```python
from build123d import *

# Parameters (mm, degrees)
CROQUIS1_R              = 3
SALIENTE_EXTRUIR1_DEPTH = 20
CROQUIS2_R              = 3
SALIENTE_EXTRUIR2_DEPTH = 3.5
REDONDEO2_R             = 1
CROQUIS3_R              = 4.296610541
CROQUIS3_R_2            = 3
SALIENTE_EXTRUIR3_DEPTH = 4.5
REDONDEO3_SIZE          = 1


with BuildPart() as part:
    # Croquis1 → Saliente-Extruir1 (new body)
    with BuildSketch(Plane.XY):
        Circle(CROQUIS1_R)
    extrude(amount=SALIENTE_EXTRUIR1_DEPTH)

    # Croquis2 → Saliente-Extruir2 (add, symmetric)
    with BuildSketch(Plane(origin=(0, 0, 0), x_dir=(1, 0, 0), z_dir=(0, 1, 0))):
        with BuildLine():
            Line((-5.504587156, -21.651376147), (-3, -20))
            Line((-3, -20), (3, -20))
            Line((3, -20), (5.504587156, -21.651376147))
            ThreePointArc((5.504587156, -21.651376147), (0, -40), (-5.504587156, -21.651376147))
        make_face()
        with Locations(Location((0, -30, 0), (0, 0, 90))):
            Circle(CROQUIS2_R, mode=Mode.SUBTRACT)
    extrude(amount=SALIENTE_EXTRUIR2_DEPTH, both=True)

    # Redondeo2
    redondeo2_edges = [part.edges().sort_by_distance(p)[0] for p in [
        (0, 3.5, 40),
        (4.252293578, 3.5, 20.825688073),
        (-4.252293578, 3.5, 20.825688073),
        (0, -3.5, 40),
        (4.252293578, -3.5, 20.825688073),
        (-4.252293578, -3.5, 20.825688073),
    ]]
    fillet(redondeo2_edges, radius=REDONDEO2_R)

    # Croquis3 → Saliente-Extruir3 (add, symmetric)
    with BuildSketch(Plane(origin=(0, 0, 0), x_dir=(1, 0, 0), z_dir=(0, 1, 0))):
        with Locations(Location((0, -30, 0), (0, 0, 270))):
            Circle(CROQUIS3_R)
        with Locations(Location((0, -30, 0), (0, 0, 90))):
            Circle(CROQUIS3_R_2, mode=Mode.SUBTRACT)
    extrude(amount=SALIENTE_EXTRUIR3_DEPTH, both=True)

    # Redondeo3
    # a fillet whose section is not a circle: 1 mm, written as the material it takes off along each edge
    with BuildSketch(Plane(origin=(0, -4.5, 30), x_dir=(0, 0, 1), z_dir=(-1, 0, 0))) as redondeo3_piece_1:
        with BuildLine():
            Bezier((4.296610541 - REDONDEO3_SIZE, 0), (4.296610541, 0), (4.296610541, REDONDEO3_SIZE), weights=[1, 0.353553391, 1])
            Line((4.296610541, REDONDEO3_SIZE), (4.296610541, 0))
            Line((4.296610541, 0), (4.296610541 - REDONDEO3_SIZE, 0))
        make_face()
    revolve(axis=Axis((0, -4.5, 30), (0, 1, 0)), mode=Mode.SUBTRACT)
    with BuildSketch(Plane(origin=(0, 4.5, 30), x_dir=(0, 0, 1), z_dir=(-1, 0, 0))) as redondeo3_piece_2:
        with BuildLine():
            Bezier((4.296610541, -REDONDEO3_SIZE), (4.296610541, 0), (4.296610541 - REDONDEO3_SIZE, 0), weights=[1, 0.353553391, 1])
            Line((4.296610541 - REDONDEO3_SIZE, 0), (4.296610541, 0))
            Line((4.296610541, 0), (4.296610541, -REDONDEO3_SIZE))
        make_face()
    revolve(axis=Axis((0, 4.5, 30), (0, 1, 0)), mode=Mode.SUBTRACT)


solid = part.part
```
Read the model definition and answer for the solid it produces. Units are mm, in the model's axes. A direction names the side the tool comes from. Give positions to 0.01 mm unless a question says otherwise; leave off trailing zeros. Loops run counter-clockwise (first coordinate to the right, second up) from the corner with the lowest first, then second, coordinate; pieces in that order, holes last.
Item 1: The mould has two halves that part along X. Classify faces 4 (the cylindrical face through (3.91, -3.2, 20.94)), 5 (the flat face through (0, 0, 0)), 6 (the cylindrical face through (0, 0, 33)), 7 (the cylindrical face through (-3, 0, 10)): released by +X, released by -X, zero draft, split by the parting line, or undercut.
Item 2: Each of these flat-tipped pins is pushed along its axis until it touches: pin 1 Ø4 at (y, z) = (1, 24) entering from +X; pin 2 Ø1.5 at (y, z) = (-1, 5) entering from +X; pin 3 Ø5.5 at (x, z) = (-2, 30) entering from +Y; pin 4 Ø6 at (x, z) = (-3, 18.5) entering from -Y. Where does it stop, or does it pass through?
Item 3: The part is cut by section B-B (y = -1). Write down the section's boundary in (x, z), and give its area (3 significant figures).
Item 4: For faces 1 (the flat face through (4, -3.5, 27)), 2 (the flat face through (-0.2, 3.2, 20)), 3 (the flat face through (-0.2, -3.2, 20)), determine the directions among +Z, -Z, +X, -X, +Y, -Y from which every point of the face is accessible in a straight line to the end or side of a thin tool.
Item 5: Find the intervals of material crossed by line 1 along X through (y, z) = (1.25, 30); line 2 along Z through (x, y) = (-1.5, -1.5); line 3 along Y through (x, z) = (-3, 23.5), in increasing order.
Item 6: The part is cut by section C-C (z = 4.5). Write down the section's boundary in (x, y).
Item 7: The part is cut by section A-A (y = 2). Write down the section's boundary in (x, z), and give its area (3 significant figures).
Taken from the geometry:
1. face 4: released by +X
1. face 5: zero draft
1. face 6: undercut
1. face 7: split by the parting line
2. pin 1: stops at x = 9.17
2. pin 2: stops at x = 2.99
2. pin 3: stops at y = 4.5
2. pin 4: stops at y = -3.5
3. outline: (-5.5, 21.65) - (-3, 20) - (-2.83, 20) - (-2.83, 0) - (2.83, 0) - (2.83, 20) - (3, 20) - (5.5, 21.65) arc R10 ccw (long way) to start; hole circle Ø6 at (0, 30)
3. area: 401 mm2
4. face 1: -Y
4. face 2: -Z, +Y
4. face 3: -Z, -Y
5. line 1: x = -10 to -3, 3 to 10
5. line 2: z = 0 to 27.4, 32.6 to 39.89
5. line 3: y = -3.5 to 3.5
6. outline: circle Ø6 at (0, 0)
7. outline: (-5.5, 21.65) - (-3, 20) - (-2.24, 20) - (-2.24, 0) - (2.24, 0) - (2.24, 20) - (3, 20) - (5.5, 21.65) arc R10 ccw (long way) to start; hole circle Ø6 at (0, 30)
7. area: 377 mm2
